Autodesk Inventor part; units mm, degrees
ref_plane "YZ Plane" through (0, 0, 0) normal (1, 0, 0) x (0, 1, 0)
ref_plane "XZ Plane" through (0, 0, 0) normal (0, 1, 0) x (-1, 0, 0)
ref_plane "XY Plane" through (0, 0, 0) normal (0, 0, 1) x (1, 0, 0)
sketch "스케치1" plane through (0, 0, 0) normal (0, 1, 0) x (-1, 0, 0)
  line L0 (0, 0) -> (40.6, 0)
  line L1 (40.6, 0) -> (40.6, -61.6)
  line L2 (40.6, -61.6) -> (0, -61.6)
  line L3 (0, -61.6) -> (0, 0)
  line L4 (42.6, -63.6) -> (42.6, 2)
  line L5 (42.6, 2) -> (-2, 2)
  line L6 (-2, 2) -> (-2, -63.6)
  line L7 (-2, -63.6) -> (42.6, -63.6)
  line L8 (35.6, 0) -> (40.6, -8)
  line L9 (40.6, -30.8) -> (0, -30.8) construction
  line L10 (20.3, 0) -> (20.3, -61.6) construction
  line L11 (35.6, -61.6) -> (40.6, -53.6)
  line L12 (0, 0) -> (0, -61.6)
  line L13 (5, 0) -> (0, -8)
  line L14 (5, -61.6) -> (0, -53.6)
  point P0 (0, -8)
  point P1 (5, 0)
  point P2 (40.6, -53.6)
  point P3 (0, -53.6)
  dimension "d0" = 40.6
  dimension "d1" = 61.6
  dimension "d2" = 2
  dimension "d3" = 5
  dimension "d4" = 8
extrude "돌출1" add sketch "스케치1" along normal blind 7 contours L0 L13 L3 | L0 L1 L8 | L14 L2 L3 | L1 L2 L11 | L7 L6 L5 L4
sketch "스케치2" plane through (0, 0, 0) normal (0, -1, 0) x (1, 0, 0)
  line L0 (-42.6, 2) -> (2, 2)
  line L1 (-42.6, -63.6) -> (-42.6, 2)
  line L2 (2, -63.6) -> (-42.6, -63.6)
  line L3 (2, 2) -> (2, -63.6)
  line L4 (0, -53.6) -> (0, -8)
  line L5 (-5, -61.6) -> (0, -53.6)
  line L6 (-35.6, -61.6) -> (-5, -61.6)
  line L7 (-40.6, -53.6) -> (-35.6, -61.6)
  line L8 (-40.6, -8) -> (-40.6, -53.6)
  line L9 (-35.6, 0) -> (-40.6, -8)
  line L10 (-5, 0) -> (-35.6, 0)
  line L11 (0, -8) -> (-5, 0)
  point P0 (0, 0)
extrude "돌출2" add sketch "스케치2" along normal blind 1 contours L0 L3 L2 L1 | L5 L6 L7 L8 L9 L10 L11 L4
sketch "스케치3" plane through (0, 0, 0) normal (0, 1, 0) x (1, 0, 0)
  line L0 (-42.6, -2) -> (2, -2)
  line L1 (2, -2) -> (2, 63.6)
  line L2 (2, 63.6) -> (-42.6, 63.6)
  line L3 (-42.6, 63.6) -> (-42.6, -2)
  line L4 (0, 53.6) -> (0, 8)
  line L5 (0, 8) -> (-5, 0)
  line L6 (-5, 0) -> (-35.6, 0)
  line L7 (-35.6, 0) -> (-40.6, 8)
  line L8 (-40.6, 8) -> (-40.6, 53.6)
  line L9 (-40.6, 53.6) -> (-35.6, 61.6)
  line L10 (-35.6, 61.6) -> (-5, 61.6)
  line L11 (-5, 61.6) -> (0, 53.6)
  line L12 (-35.1, 61.6) -> (-5.5, 61.6)
  line L13 (-5.5, 61.6) -> (-5.5, 5.5)
  line L14 (-5.5, 5.5) -> (-35.1, 5.5)
  line L15 (-35.1, 5.5) -> (-35.1, 61.6)
  line L16 (-35.6, 61.6) -> (-5, 61.6)
  point P0 (0, 0)
  dimension "d9" = 5.5
  dimension "d10" = 5.5
  dimension "d11" = 5.5
extrude "돌출3" add sketch "스케치3" along normal blind 3 contours L4 L5 L6 L7 L8 L9 L10 L15 L14 L13 L11
sketch "스케치4" plane through (0, 0, 0) normal (0, 1, 0) x (1, 0, 0)
  line L0 (-5.5, 5.5) -> (-5.5, 61.6)
  line L1 (-35.1, 61.6) -> (-5.5, 61.6)
  line L2 (-35.1, 61.6) -> (-35.1, 5.5)
  line L3 (-35.1, 5.5) -> (-5.5, 5.5)
  circle A0 centre (-20.3, 48.6) radius 4.5
  point P0 (0, 0)
  dimension "d15" = 9
  dimension "d18" = 13
extrude "돌출4" cut sketch "스케치4" against normal blind 7 contours A0
sketch "스케치5" plane through (0, 3, 0) normal (0, 1, 0) x (1, 0, 0)
  line L0 (-42.6, -2) -> (2, -2)
  line L1 (-40.6, 8) -> (-40.6, 53.6)
  line L2 (-35.6, 0) -> (-40.6, 8)
  line L3 (-5, 0) -> (-35.6, 0)
  line L4 (0, 8) -> (-5, 0)
  line L5 (0, 53.6) -> (0, 8)
  line L6 (-5, 61.6) -> (0, 53.6)
  line L7 (-5.5, 61.6) -> (-5, 61.6)
  line L8 (-5.5, 61.6) -> (-5.5, 5.5)
  line L9 (-5.5, 5.5) -> (-35.1, 5.5)
  line L10 (-35.1, 5.5) -> (-35.1, 61.6)
  line L11 (-35.6, 61.6) -> (-35.1, 61.6)
  line L12 (-40.6, 53.6) -> (-35.6, 61.6)
  line L13 (-37.6, 4.5) -> (-37.6, 58.8776) construction
  circle A0 centre (-37.6, 53.6) radius 1.35
  line L14 (2, 63.6) -> (-42.6, 63.6) construction
  circle A1 centre (-37.6, 31.2) radius 1.35
  circle A2 centre (-37.6, 8.8) radius 1.35
  line L15 (-20.3, 5.5) -> (-20.3, 61.6) construction
  line L16 (-35.6, 61.6) -> (-5, 61.6) construction
  line L17 (-5, 0) -> (0, 8)
  line L18 (-5.5, 5.5) -> (-5.5, 61.6)
  circle A3 centre (-3, 53.6) radius 1.35
  circle A4 centre (-3, 31.2) radius 1.35
  circle A5 centre (-3, 8.8) radius 1.35
  point P0 (0, 0)
  dimension "d20" = 2.7
  dimension "d21" = 10
  dimension "d24" = 22.4
  dimension "d31" = 34.6
extrude "돌출5" cut sketch "스케치5" against normal through all contours A0 | A1 | A2 | A3 | A4 | A5
properties part number "mx-64"
Source: CAD feature listing. Evaluate the final solid. Frame: model axes, mm. A direction names the side the tool comes from. Give positions to 0.01 mm unless a question says otherwise; leave off trailing zeros. Write each loop counter-clockwise with the first axis right and the second up, starting at its lowest first coordinate (ties: lowest second). Pieces come first, ordered by that corner, then holes. Notation, with made-up numbers: M 3,-11 L 57,-11 A20 ccw 57,19 Z; hole C -4.5,77.5 d11. An arc over 180 degrees is marked long. Return JSON: item names as keys, results as strings. Group by question number.
1) Pin query (flat end, axial travel): P1, Ø8, axis at x = -20.3, z = -48.6, coming from the +Y side; P2, Ø3.5, axis at x = -37.6, z = -31.2, coming from the +Y side. Return the tip coordinate at first contact, or that it passes through.
2) Cut plane A-A, the plane x = -37.6. Output: boundary loops of the cut face in (y, z), plus the area to 3 significant figures.
3) Cut plane D-D, the plane z = -33.5. Output: boundary loops of the cut face in (x, y), plus the area to 3 significant figures.
4) Cut plane B-B, the plane x = -20.3. Output: boundary loops of the cut face in (y, z), plus the area to 3 significant figures.
5) Set-up query: faces 4 (the face through (-36.353, 1.028, -8.283)), 5 (the face through (-2.535, 4.972, -57.656)). Return all of +Z, -Z, +X, -X, +Y, -Y with unobstructed straight access to the full face (end or side cutting, diameter ignored); none if empty.
6) Cut plane C-C, the plane y = 4. Output: boundary loops of the cut face in (x, z).
7) Pull-direction query (Z, two-part tool) for faces 1 (the face through (-21, -1, -30)), 2 (the face through (-21, 3, 2)), 3 (the face through (-20, 5, 0)); classes: pulls with the +Z half, pulls with the -Z half, needs draft (parallel to the pull), parting line crosses it, or undercut.
8) Material intervals for line 1 along Z through (x, y) = (-3, -0.1); line 2 along X through (y, z) = (1.1, -31.2); line 3 along X through (y, z) = (1.75, -44.5), sorted ascending. Write a range as [from, to].
Recorded:
{
 "1": {"P1": "passes through", "P2": "stops at y = 3"},
 "2": {"outline": "M -1,-63.6 L 7,-63.6 L 7,-58.4 L 3,-58.4 L 3,-54.95 L -1,-54.95 Z; M -1,-52.25 L 3,-52.25 L 3,-32.55 L -1,-32.55 Z; M -1,-29.85 L 3,-29.85 L 3,-10.15 L -1,-10.15 Z; M -1,-7.45 L 3,-7.45 L 3,-3.2 L 7,-3.2 L 7,2 L -1,2 Z", "area": "272 mm²"},
 "3": {"outline": "M -42.6,-1 L 2,-1 L 2,7 L 0,7 L 0,3 L -5.5,3 L -5.5,0 L -35.1,0 L -35.1,3 L -40.6,3 L -40.6,7 L -42.6,7 Z", "area": "106 mm²"},
 "4": {"outline": "M -1,-63.6 L 7,-63.6 L 7,-61.6 L 0,-61.6 L 0,-53.1 L -1,-53.1 Z; M -1,-44.1 L 0,-44.1 L 0,-5.5 L 3,-5.5 L 3,0 L 7,0 L 7,2 L -1,2 Z", "area": "101 mm²"},
 "5": {"face 4": "+Y, -Y", "face 5": "+Y"},
 "6": {"outline": "M -42.6,-63.6 L 2,-63.6 L 2,2 L -42.6,2 Z; hole M -40.6,-53.6 L -35.6,-61.6 L -5,-61.6 L 0,-53.6 L 0,-8 L -5,0 L -35.6,0 L -40.6,-8 Z"},
 "7": {"face 1": "needs draft", "face 2": "pulls with the +Z half", "face 3": "undercut"},
 "8": {"line 1": "z = [-63.6, -54.95], [-52.25, -32.55], [-29.85, -10.15], [-7.45, 2]", "line 2": "x = [-42.6, -38.95], [-36.25, -35.1], [-5.5, -4.35], [-1.65, 2]", "line 3": "x = [-42.6, -35.1], [-5.5, 2]"}
}
